Source: CAD feature listing. Evaluate the final solid. Frame: model axes, mm. Face numbers are marked on the shaded views. A direction names the side the tool comes from. Give positions to 0.01 mm unless a question says otherwise; leave off trailing zeros. Write each loop counter-clockwise with the first axis right and the second up, starting at its lowest first coordinate (ties: lowest second). Pieces come first, ordered by that corner, then holes. Notation, with made-up numbers: (-38, -27) -> (-27, -27) arc R26 cw to (-27, 7) -> close; hole circle Ø7 at (2, 86). An arc over 180 degrees is marked (long way). Use a Markdown table: item, result. Add a question column.
```python
from build123d import *

# Parameters (mm, degrees)
CROQUIS1_R              = 13.5
SALIENTE_EXTRUIR1_DEPTH = 5
CROQUIS2_R              = 10
CORTAR_EXTRUIR1_DEPTH   = 1
CORTAR_EXTRUIR2_START   = -1
CROQUIS3_R              = 10
CORTAR_EXTRUIR2_DEPTH   = 1
CROQUIS4_R              = 5
SALIENTE_EXTRUIR2_DEPTH = 4
CROQUIS5_R              = 4
CORTAR_EXTRUIR4_DEPTH   = 21.700241544


with BuildPart() as part:
    # Croquis1 → Saliente-Extruir1 (new body)
    with BuildSketch(Plane(origin=(0, 0, 0), x_dir=(0, 0, -1), z_dir=(1, 0, 0))):
        Circle(CROQUIS1_R)
    extrude(amount=SALIENTE_EXTRUIR1_DEPTH)

    # Croquis2 → Cortar-Extruir1 (cut)
    with BuildSketch(Plane(origin=(5, 0, 0), x_dir=(0, 0, -1), z_dir=(1, 0, 0))):
        Circle(CROQUIS2_R)
    extrude(amount=-CORTAR_EXTRUIR1_DEPTH, mode=Mode.SUBTRACT)

    # Croquis3 → Cortar-Extruir2 (cut)
    with BuildSketch(Plane.ZY.offset(CORTAR_EXTRUIR2_START)):
        with Locations(Location((0, 0, 0), (0, 0, 180))):
            Circle(CROQUIS3_R)
    extrude(amount=CORTAR_EXTRUIR2_DEPTH, mode=Mode.SUBTRACT)

    # Croquis4 → Saliente-Extruir2 (add)
    with BuildSketch(Plane(origin=(4, 0, 0), x_dir=(0, 0, -1), z_dir=(1, 0, 0))):
        Circle(CROQUIS4_R)
    extrude(amount=SALIENTE_EXTRUIR2_DEPTH)

    # Croquis5 → Cortar-Extruir4 (cut, through all)
    with BuildSketch(Plane(origin=(8, 0, 0), x_dir=(0, 0, -1), z_dir=(1, 0, 0))):
        Circle(CROQUIS5_R)
    extrude(amount=-CORTAR_EXTRUIR4_DEPTH, mode=Mode.SUBTRACT)


solid = part.part
```
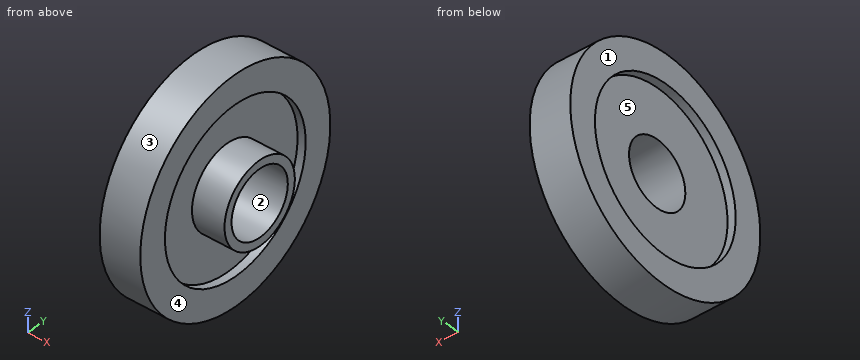
(1) Mould query, pull axis Y, two halves, no side actions, for the marked faces 1, 2 and 3. Classes: +Y half, -Y half, draft (parallel to the pull), parting line (faces both ways), or undercut.
(2) First-contact query: pin 1 Ø16 at (y, z) = (-1, -0.5) entering from -X; pin 2 Ø4 at (x, y) = (1.5, -5.5) entering from -Z; pin 3 Ø3 at (x, y) = (3.5, -6) entering from -Z. Flat tips, straight axial feed; report the tip coordinate or a pass-through.
(3) Cut plane D-D on z = 10.5. Return the cut outline in (x, y).
(4) Material intervals for L1, parallel to Y at x = 4.35, z = 0; L2, parallel to Y at x = 0.35, z = 0; L3, parallel to Y at x = 4.25, z = -1, sorted ascending.
(5) Cut plane A-A on z = 0. Return the cut outline in (x, y).
(6) Access query for the marked faces 4 and 5. Directions: +Z, -Z, +X, -X, +Y, -Y. A direction counts if a zero-diameter tool reaches every point of the face in a straight line with its end or side. Return the directions, or none.
(7) Cut plane C-C on x = 6. Return the cut outline in (y, z), then the cut area to 3 significant figures.
Output:
| question | item | result |
|---|---|---|
| 1 | face 1 | draft |
| 1 | face 2 | undercut |
| 1 | face 3 | parting line |
| 2 | pin 1 | x = 1 |
| 2 | pin 2 | z = -13.04 |
| 2 | pin 3 | z = -12.73 |
| 3 | outline | (0, -8.49) -> (5, -8.49) -> (5, 8.49) -> (0, 8.49) -> close |
| 4 | L1 | -13.5 to -10, -5 to -4, 4 to 5, 10 to 13.5 |
| 4 | L2 | -13.5 to -10, 10 to 13.5 |
| 4 | L3 | -13.46 to -9.95, -4.9 to -3.87, 3.87 to 4.9, 9.95 to 13.46 |
| 5 | outline | (0, -13.5) -> (5, -13.5) -> (5, -10) -> (4, -10) -> (4, -5) -> (8, -5) -> (8, -4) -> (1, -4) -> (1, -10) -> (0, -10) -> close; (0, 10) -> (1, 10) -> (1, 4) -> (8, 4) -> (8, 5) -> (4, 5) -> (4, 10) -> (5, 10) -> (5, 13.5) -> (0, 13.5) -> close |
| 6 | face 4 | +X |
| 6 | face 5 | -X |
| 7 | outline | circle Ø10 at (0, 0); hole circle Ø8 at (0, 0) |
| 7 | area | 28.3 mm^2 |
